Geometry: final body of the model. Coordinates: model frame, mm. Face numbers are marked on the shaded views. Give positions to 0.01 mm unless a question says otherwise; leave off trailing zeros. Write each loop counter-clockwise with the first axis right and the second up, starting at its lowest first coordinate (ties: lowest second). Pieces come first, ordered by that corner, then holes. Notation, with made-up numbers: M 75.25,33 L 113.25,33 A21 cw 113.25,52 Z; hole C 41,11 d1. An arc over 180 degrees is marked long. Use one line per item in the form item = value. Start each with the question number.
Item 1: Material intervals for line 1 along X through (y, z) = (200, -19); line 2 along Y through (x, z) = (0, -25); line 3 along Y through (x, z) = (2.5, -23), sorted ascending. Write a range as from..to.
Item 2: Section query C-C on y = 203. Return loops of the section in (x, z), then the cut area to 3 significant figures.
Item 3: Section query B-B on z = -9.5. Return loops of the section in (x, y).
Item 4: Pull-direction query (Y, two-part tool) for the marked faces 1, 2 and 3; classes: released by +Y, released by -Y, zero draft, split by the parting line, or undercut.
Item 5: Contact query for flat-ended pins moving along their axis: P1, Ø6, axis at x = -12.5, z = -27, coming from the +Y side; P2, Ø10, axis at x = -1.5, y = 189.5, coming from the -Z side; P3, Ø3, axis at y = 210, z = -18, coming from the -X side. Output: stop coordinate, or through.
Item 6: Section query D-D on z = -29. Return loops of the section in (x, y), then the cut area to 3 significant figures.
Item 7: Section query A-A on x = 0. Return loops of the section in (y, z).
from build123d import *

# Parameters (mm, degrees)
SKETCH1_R           = 17.15
SKETCH1_R_2         = 16.15
BOSS_EXTRUDE1_DEPTH = 40
BOSS_EXTRUDE2_DEPTH = 40
SKETCH2_R           = 18
CUT_EXTRUDE1_DEPTH  = 369.15


with BuildPart() as part:
    # Sketch1 → Boss-Extrude1 (new body)
    with BuildSketch(Plane.XY):
        with Locations((0, 200)):
            Circle(SKETCH1_R)
        with Locations((0, 200)):
            Circle(SKETCH1_R_2, mode=Mode.SUBTRACT)
    extrude(amount=-BOSS_EXTRUDE1_DEPTH)

    # Sketch3 → Boss-Extrude2 (add)
    with BuildSketch(Plane(origin=(0, 0, -40), x_dir=(-1, 0, 0), z_dir=(0, 0, -1))):
        Polygon((17.15, 182.85), (17.15, 181.85), (-17.15, 181.85), (-17.15, 182.85), (0, 182.85), align=None)
        with BuildLine():
            Line((17.15, 182.85), (17.15, 200))
            ThreePointArc((17.15, 200), (12.126881297, 187.873118703), (0, 182.85))
            Line((0, 182.85), (17.15, 182.85))
        make_face()
        with BuildLine():
            ThreePointArc((0, 182.85), (-12.126881297, 187.873118703), (-17.15, 200))
            Line((-17.15, 200), (-17.15, 182.85))
            Line((-17.15, 182.85), (0, 182.85))
        make_face()
    extrude(amount=-BOSS_EXTRUDE2_DEPTH)

    # Sketch2 → Cut-Extrude1 (cut, through all)
    with BuildSketch(Plane(origin=(0, 550, 0), x_dir=(1, 0, 0), z_dir=(0, 1, 0))):
        Circle(SKETCH2_R)
    extrude(amount=-CUT_EXTRUDE1_DEPTH, mode=Mode.SUBTRACT)


solid = part.part
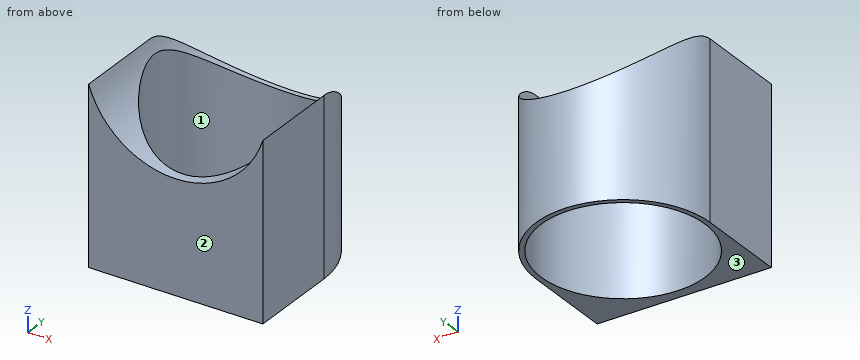
Answer sheet:
q1.line_1 = -17.15..-16.15, 16.15..17.15
q1.line_2 = 181.85..183.85, 216.15..217.15
q1.line_3 = 181.85..184.04, 215.96..216.97
q2.outline = M -16.89,-40 L -15.87,-40 L -15.87,-8.5 A18 cw -16.89,-6.24 Z; M 15.87,-40 L 16.89,-40 L 16.89,-6.24 A18 cw 15.87,-8.5 Z
q2.area = 66.2 mm2
q3.outline = M -17.15,181.85 L -15.29,181.85 L -15.29,194.8 A16.15 cw -15.29,205.2 L -15.29,207.77 A17.15 ccw -17.15,200 Z; M 15.29,181.85 L 17.15,181.85 L 17.15,200 A17.15 ccw 15.29,207.77 L 15.29,205.2 A16.15 cw 15.29,194.8 Z
q4.face_1 = undercut
q4.face_2 = released by -Y
q4.face_3 = zero draft
q5.P1 = 214.28
q5.P2 = through
q5.P3 = -14.9
q6.outline = M -17.15,181.85 L 17.15,181.85 L 17.15,200 A17.15 ccw -17.15,200 Z; hole C 0,200 d32.3
q6.area = 265 mm2
q7.outline = M 181.85,-40 L 183.85,-40 L 183.85,-18 L 181.85,-18 Z; M 216.15,-40 L 217.15,-40 L 217.15,-18 L 216.15,-18 Z
